Autodesk Inventor part; units mm, degrees
ref_plane "YZ Plane" through (0, 0, 0) normal (1, 0, 0) x (0, 1, 0)
ref_plane "XZ Plane" through (0, 0, 0) normal (0, 1, 0) x (-1, 0, 0)
ref_plane "XY Plane" through (0, 0, 0) normal (0, 0, 1) x (1, 0, 0)
sketch "Sketch1" plane through (0, 0, 0) normal (0, 1, 0) x (-1, 0, 0)
  line L0 (0, 0) -> (38.1, 0)
  line L1 (38.1, 0) -> (38.1, -101.6)
  line L2 (38.1, -101.6) -> (0, -101.6)
  line L3 (0, -101.6) -> (0, 0)
  line L4 (38.1, -101.6) -> (32.385, -101.6)
  line L5 (32.385, -101.6) -> (32.385, 0)
  line L6 (32.385, 0) -> (38.1, 0)
  line L7 (38.1, 0) -> (38.1, -101.6)
  line L8 (0, -101.6) -> (5.715, -101.6)
  line L9 (5.715, -101.6) -> (5.715, 0)
  line L10 (5.715, 0) -> (0, 0)
  line L11 (0, 0) -> (0, -101.6)
  dimension "d0" = 38.1
  dimension "d1" = 101.6
  dimension "d2" = 5.715
  dimension "d3" = 5.715
extrude "Extrusion1" add sketch "Sketch1" along normal blind 25.4 contours L0 L9 L2 L3 | L0 L1 L2 L5
extrude "Extrusion2" add sketch "Sketch1" against normal blind 5.08
sketch "Sketch2" plane through (0, 25.4, 0) normal (1, 0, 0) x (0, 0, -1)
  line L0 (101.6, 0) -> (0, 0)
  line L1 (50.8, 0) -> (50.8, -12.7)
  point P0 (0, -25.4)
  dimension "d8" = 12.7
hole "Hole1" at (0, 12.7, -50.8) direction (-1, 0, 0) diameter 6.7564 end through all
sketch "Sketch3" plane through (0, -5.08, 0) normal (0, -1, 0) x (1, 0, 0)
  line L0 (0, 0) -> (0, -101.6)
  line L1 (0, 0) -> (-6.223, 0)
  line L2 (-6.223, 0) -> (-6.223, -101.6)
  line L3 (-6.223, -101.6) -> (0, -101.6)
  line L4 (0, -101.6) -> (0, 0)
  line L5 (-38.1, -101.6) -> (-38.1, 0)
  line L6 (-38.1, 0) -> (-31.877, 0)
  line L7 (-31.877, 0) -> (-31.877, -101.6)
  line L8 (-31.877, -101.6) -> (-38.1, -101.6)
  line L9 (-38.1, -101.6) -> (-38.1, 0)
  dimension "d16" = 6.223
  dimension "d17" = 101.6
  dimension "d18" = 6.223
extrude "Extrusion3" add sketch "Sketch3" along normal blind 12.7
sketch "Sketch4" plane through (-38.1, 25.4, -101.6) normal (-1, 0, 0) x (0, 0, 1)
  line L0 (101.6, -43.18) -> (101.6, 0)
  line L1 (101.6, -43.18) -> (88.9, -43.18)
  line L2 (88.9, -43.18) -> (88.9, -36.83)
  line L3 (88.9, -36.83) -> (101.6, -36.83)
  line L4 (101.6, -36.83) -> (101.6, -43.18)
  line L5 (0, -43.18) -> (0, 0)
  line L6 (0, -43.18) -> (12.7, -43.18)
  line L7 (12.7, -43.18) -> (12.7, -36.83)
  line L8 (12.7, -36.83) -> (0, -36.83)
  line L9 (0, -36.83) -> (0, -43.18)
  point P0 (101.6, -25.4)
  dimension "d21" = 12.7
  dimension "d22" = 6.35
  dimension "d23" = 12.7
hole "Hole2" at (-38.1, -11.43, -12.7) at (-38.1, -11.43, -88.9) direction (1, 0, 0) diameter 6.7564 end through all
fillet "Fillet1" radius 3.175 6 edges at (-38.1, 3.81, 0) (-38.1, 25.4, -50.8) (0, 3.81, 0) (0, 25.4, -50.8) (0, 3.81, -101.6) (-38.1, 3.81, -101.6)
sketch "Sketch5" plane through (0, -17.78, -98.425) normal (1, 0, 0) x (0, 0, -1)
  line L0 (-95.25, 0) -> (0, 0)
  line L1 (-47.625, 0) -> (-47.625, 17.78)
  line L2 (-47.625, 17.78) -> (-47.625, 8.89)
  line L3 (-98.425, 17.78) -> (3.175, 17.78)
  line L4 (-73.025, 0) -> (-22.225, 0)
  line L5 (-22.225, 0) -> (-22.225, 17.78)
  line L6 (-22.225, 17.78) -> (-73.025, 17.78)
  line L7 (-73.025, 17.78) -> (-73.025, 0)
  line L8 (-73.025, 0) -> (-22.225, 17.78) construction
  line L9 (-22.225, 0) -> (-73.025, 17.78) construction
  dimension "d32" = 50.8
extrude "Extrusion4" cut sketch "Sketch5" against normal blind 25.4
properties part number "Rail Clip"
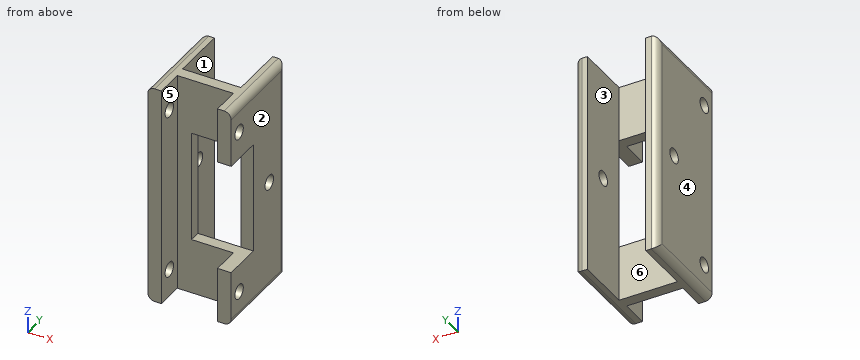
The model under review builds one solid part; all positions refer to its coordinate system, in mm. Face numbers are marked on the shaded views. A direction names the side the tool comes from. Round coordinates to 2 decimals unless told otherwise and drop trailing zeros. Loops run counter-clockwise (first coordinate to the right, second up) from the corner with the lowest first, then second, coordinate; pieces in that order, holes last. Notation, with made-up numbers: (10.5, -13) -> (44.5, -13) arc R22 ccw to (44.5, 23) -> close; hole circle Ø8 at (72.5, 56). An arc over 180 degrees is marked (long way). Write item = value, one per line. Start each with the question number.
Item 1: Take a section at A-A on z = -28.5. Give the boundary of the cut face in (x, y) (3 decimals).
Item 2: To check wall thickness, follow L1, parallel to Z at x = -4, y = -11.43; L2, parallel to Z at x = -33.5, y = -11.43; L3, parallel to Z at x = -4, y = -3. State the ranges of each line that lie inside material, in increasing order.
Item 3: Mouldability with a two-part tool opening along X and no side actions: class the marked faces 1, 2, 3 and 4 as released by +X, released by -X, zero draft, split by the parting line, or undercut.
Item 4: Take a section at C-C on x = -21.5. Give the boundary of the cut face in (y, z), plus the area to 3 significant figures.
Item 5: Take a section at D-D on z = -12.7. Give the boundary of the cut face in (x, y) (3 decimals), plus the area to 3 significant figures.
Item 6: For the marked faces 5 and 6, list the 3-axis set-ups (+Z, -Z, +X, -X, +Y, -Y) from which the entire face can be reached by the end or side of a thin tool; tool diameter is ignored.
Item 7: Insertion check: pin 1 (5.5 mm diameter, centred on y = -3.5, z = -53, fed in from +X); pin 2 (7.5 mm diameter, centred on x = -23, z = -35, fed in from -Y); pin 3 (8 mm diameter, centred on x = -27, z = -75, fed in from +Y). Each pin has a flat end and moves straight along its axis. Give the tip position at first contact, or say it passes through.
Item 8: Take a section at B-B on y = -6.5. Give the boundary of the cut face in (x, z) (3 decimals).
Result:
q1.outline = (-38.1, -17.78) -> (-31.877, -17.78) -> (-31.877, -5.08) -> (-25.4, -5.08) -> (-25.4, 0) -> (-32.385, 0) -> (-32.385, 25.4) -> (-34.925, 25.4) arc R3.175 ccw to (-38.1, 22.225) -> close; (-5.715, 0) -> (0, 0) -> (0, 22.225) arc R3.175 ccw to (-3.175, 25.4) -> (-5.715, 25.4) -> close
q2.L1 = -101.6 to -92.28, -85.52 to -76.2, -25.4 to -16.08, -9.32 to 0
q2.L2 = -101.6 to -92.28, -85.52 to -16.08, -9.32 to 0
q2.L3 = -101.6 to -76.2, -25.4 to 0
q3.face_1 = undercut
q3.face_2 = released by +X
q3.face_3 = undercut
q3.face_4 = released by -X
q4.outline = (-5.08, -101.6) -> (0, -101.6) -> (0, -76.2) -> (-5.08, -76.2) -> close; (-5.08, -25.4) -> (0, -25.4) -> (0, 0) -> (-5.08, 0) -> close
q4.area = 258 mm²
q5.outline = (-38.1, -17.78) -> (-31.877, -17.78) -> (-31.877, -14.808) -> (-38.1, -14.808) -> close; (-38.1, -8.052) -> (-31.877, -8.052) -> (-31.877, -5.08) -> (-6.223, -5.08) -> (-6.223, -8.052) -> (0, -8.052) -> (0, 22.225) arc R3.175 ccw to (-3.175, 25.4) -> (-5.715, 25.4) -> (-5.715, 0) -> (-32.385, 0) -> (-32.385, 25.4) -> (-34.925, 25.4) arc R3.175 ccw to (-38.1, 22.225) -> close; (-6.223, -17.78) -> (0, -17.78) -> (0, -14.808) -> (-6.223, -14.808) -> close
q5.area = 554 mm²
q6.face_5 = +Z, -Z, -Y
q6.face_6 = +Z, -Z, +Y
q7.pin_1 = -25.4
q7.pin_2 = -5.08
q7.pin_3 = 0
q8.outline = (-38.1, -98.425) arc R3.175 ccw to (-34.925, -101.6) -> (-31.877, -101.6) -> (-31.877, 0) -> (-34.925, 0) arc R3.175 ccw to (-38.1, -3.175) -> close; (-6.223, -101.6) -> (-3.175, -101.6) arc R3.175 ccw to (0, -98.425) -> (0, -76.2) -> (-6.223, -76.2) -> close; (-6.223, -25.4) -> (0, -25.4) -> (0, -3.175) arc R3.175 ccw to (-3.175, 0) -> (-6.223, 0) -> close
